```python
from build123d import *

# Parameters (mm, degrees)
F0_R     = 2.8256485239
F0_R_2   = 3.5765465122
F0_R_3   = 2.7439429232
F0_R_4   = 3.3466336439
F0_R_5   = 3.4276298102
F0_R_6   = 3.6294104123
F0_R_7   = 2.635041669
F0_R_8   = 2.702327646
F0_R_9   = 2.972249944
F0_R_10  = 2.6404432644
F0_R_11  = 2.6241403427
F0_R_12  = 2.7159497561
F0_R_13  = 2.2390207397
F0_R_14  = 2.2607819858
F0_R_15  = 1.9741758504
F0_R_16  = 2.1219308593
F0_R_17  = 1.8827842167
F0_R_18  = 1.845321618
F0_R_19  = 1.9213841029
F1_DEPTH = 25


with BuildPart() as f1:
    # F0 (on Front) → F1 (new body)
    with BuildSketch(Plane.XZ):
        with BuildLine():
            ThreePointArc((24.5960952758, -4.4757230907), (24.8988190673, -2.2469555075), (25, 0))
            ThreePointArc((25, 0), (24.9769503507, 1.073289886), (24.9078439057, 2.1446006555))
            ThreePointArc((24.9078439057, 2.1446006555), (0.5208838947, 24.9945730103), (-24.7968706797, 3.1804409279))
            ThreePointArc((-24.7968706797, 3.1804409279), (-23.1514874221, -9.4344385176), (-15.5110739298, -19.6062894384))
            ThreePointArc((-15.5110739298, -19.6062894384), (-13.7709472228, -14.2438804489), (-9.2095510788, -17.5570566207))
            ThreePointArc((-9.2095510788, -17.5570566207), (-10.6398306506, -20.3713740635), (-13.7563172666, -20.8749547368))
            ThreePointArc((-13.7563172666, -20.8749547368), (-7.1807427047, -23.9465432622), (0, -25))
            ThreePointArc((0, -25), (13.7903970721, -20.8524566561), (23.0050925772, -9.7859958876))
            ThreePointArc((23.0050925772, -9.7859958876), (16.860220208, -5.0514647504), (24.5960952758, -4.4757230907))
        make_face()
        with Locations((-7.0527321659, -21.0157949477)):
            Circle(F0_R, mode=Mode.SUBTRACT)
        with Locations((-18.0755164474, -11.404263787)):
            Circle(F0_R_2, mode=Mode.SUBTRACT)
        with Locations((-21.2986432016, -5.0265877508)):
            Circle(F0_R_3, mode=Mode.SUBTRACT)
        Polygon((4.266737029, -20.0934484601), (0, -25), (-2.6190390345, -20.0934484601), align=None, mode=Mode.SUBTRACT)
        with Locations((9.209163487, -19.5164699107)):
            Circle(F0_R_4, mode=Mode.SUBTRACT)
        with Locations((14.8604605347, -15.1914991438)):
            Circle(F0_R_5, mode=Mode.SUBTRACT)
        with BuildLine():
            Line((-18.9121421427, -0.7938772906), (-24.7968706797, 3.1804409279))
            Line((-24.7968706797, 3.1804409279), (-19.3468905014, 5.0684465431))
            ThreePointArc((-19.3468905014, 5.0684465431), (-21.9186154294, 11.469459375), (-15.5548330751, 8.8069401681))
            ThreePointArc((-15.5548330751, 8.8069401681), (-16.5182971087, 6.3016908172), (-18.9121421427, 5.0875890061))
            Line((-18.9121421427, 5.0875890061), (-18.9121421427, -0.7938772906))
        make_face(mode=Mode.SUBTRACT)
        with Locations((-7.0253848098, 20.105432719)):
            Circle(F0_R_6, mode=Mode.SUBTRACT)
        with BuildLine():
            Line((19.5046194307, 4.8279847044), (24.9078439057, 2.1446006555))
            Line((24.9078439057, 2.1446006555), (18.717167899, 0))
            Line((18.717167899, 0), (18.717167899, 4.7704775792))
            ThreePointArc((18.717167899, 4.7704775792), (17.4488389654, 5.1069570809), (16.4242905584, 5.9268212774))
            ThreePointArc((16.4242905584, 5.9268212774), (17.1998275024, 3.0083990244), (17.4609430101, 0))
            ThreePointArc((17.4609430101, 0), (-6.6059492578, -16.1631050607), (-12.4625227562, 12.2298837833))
            ThreePointArc((-12.4625227562, 12.2298837833), (-16.8312529103, 17.4566617233), (-10.3065616702, 15.4987508431))
            ThreePointArc((-10.3065616702, 15.4987508431), (-10.4242678564, 14.5913936768), (-10.7695943307, 13.7441030538))
            ThreePointArc((-10.7695943307, 13.7441030538), (-2.5101792072, 17.2795697617), (6.4137999623, 16.2403109836))
            ThreePointArc((6.4137999623, 16.2403109836), (5.9393579148, 21.9051948536), (10.9397131516, 19.2010402679))
            ThreePointArc((10.9397131516, 19.2010402679), (9.558784183, 16.551960716), (6.5962795119, 16.1670537638))
            ThreePointArc((6.5962795119, 16.1670537638), (9.4231129686, 14.6999820674), (11.9364463054, 12.7438526513))
            ThreePointArc((11.9364463054, 12.7438526513), (14.1879258767, 18.3986934482), (19.0337079573, 14.7156538442))
            ThreePointArc((19.0337079573, 14.7156538442), (17.0365778867, 11.3571292026), (13.1320353046, 11.5080050208))
            ThreePointArc((13.1320353046, 11.5080050208), (14.5572332623, 9.6421725015), (15.7192265164, 7.6020029287))
            ThreePointArc((15.7192265164, 7.6020029287), (18.7083751896, 11.1226574982), (22.0615752041, 7.9468004405))
            ThreePointArc((22.0615752041, 7.9468004405), (21.3406257649, 5.9303038237), (19.5046194307, 4.8279847044))
        make_face(mode=Mode.SUBTRACT)
        Polygon((3.975788597, 19.6694843471), (-2.6190390345, 19.6694843471), (0, 24.2276750505), align=None, mode=Mode.SUBTRACT)
        with BuildLine():
            ThreePointArc((23.0050925772, -9.7859958876), (23.9482362722, -7.1750943862), (24.5960952758, -4.4757230907))
            ThreePointArc((24.5960952758, -4.4757230907), (16.860220208, -5.0514647504), (23.0050925772, -9.7859958876))
        make_face()
        with Locations((20.8382867277, -6.2433271669)):
            Circle(F0_R_7, mode=Mode.SUBTRACT)
        with BuildLine():
            ThreePointArc((11.9364463054, 12.7438526513), (12.5494630323, 12.1406551883), (13.1320353046, 11.5080050208))
            ThreePointArc((13.1320353046, 11.5080050208), (17.0365778867, 11.3571292026), (19.0337079573, 14.7156538442))
            ThreePointArc((19.0337079573, 14.7156538442), (14.1879258767, 18.3986934482), (11.9364463054, 12.7438526513))
        make_face()
        with Locations((15.2111686766, 14.7156538442)):
            Circle(F0_R_8, mode=Mode.SUBTRACT)
        with BuildLine():
            ThreePointArc((-15.5548330751, 8.8069401681), (-21.9186154294, 11.469459375), (-19.3468905014, 5.0684465431))
            Line((-19.3468905014, 5.0684465431), (-18.9121421427, 5.2190539427))
            Line((-18.9121421427, 5.2190539427), (-18.9121421427, 5.0875890061))
            ThreePointArc((-18.9121421427, 5.0875890061), (-16.5182971087, 6.3016908172), (-15.5548330751, 8.8069401681))
        make_face()
        with Locations((-19.2937050015, 8.8069401681)):
            Circle(F0_R_9, mode=Mode.SUBTRACT)
        with Locations((-7.0253848098, 20.105432719)):
            Circle(F0_R_6)
        with Locations((-7.0253848098, 20.105432719)):
            Circle(F0_R_10, mode=Mode.SUBTRACT)
        with Locations((-18.0755164474, -11.404263787)):
            Circle(F0_R_2)
        with Locations((-18.0755164474, -11.404263787)):
            Circle(F0_R_11, mode=Mode.SUBTRACT)
        with BuildLine():
            ThreePointArc((-10.3065616702, 15.4987508431), (-16.8312529103, 17.4566617233), (-12.4625227562, 12.2298837833))
            ThreePointArc((-12.4625227562, 12.2298837833), (-11.6407057812, 13.0145495395), (-10.7695943307, 13.7441030538))
            ThreePointArc((-10.7695943307, 13.7441030538), (-10.4242678564, 14.5913936768), (-10.3065616702, 15.4987508431))
        make_face()
        with Locations((-13.8626694679, 15.4987508431)):
            Circle(F0_R_12, mode=Mode.SUBTRACT)
        with BuildLine():
            ThreePointArc((-9.2095510788, -17.5570566207), (-13.7709472228, -14.2438804489), (-15.5110739298, -19.6062894384))
            ThreePointArc((-15.5110739298, -19.6062894384), (-14.6474374814, -20.2596291977), (-13.7563172666, -20.8749547368))
            ThreePointArc((-13.7563172666, -20.8749547368), (-10.6398306506, -20.3713740635), (-9.2095510788, -17.5570566207))
        make_face()
        with Locations((-12.6935141161, -17.5570566207)):
            Circle(F0_R_13, mode=Mode.SUBTRACT)
        with Locations((14.8604605347, -15.1914991438)):
            Circle(F0_R_5)
        with Locations((14.8604605347, -15.1914991438)):
            Circle(F0_R_14, mode=Mode.SUBTRACT)
        with Locations((9.209163487, -19.5164699107)):
            Circle(F0_R_4)
        with Locations((9.209163487, -19.5164699107)):
            Circle(F0_R_15, mode=Mode.SUBTRACT)
        with BuildLine():
            ThreePointArc((6.4137999623, 16.2403109836), (6.5051428606, 16.2039392484), (6.5962795119, 16.1670537638))
            ThreePointArc((6.5962795119, 16.1670537638), (9.558784183, 16.551960716), (10.9397131516, 19.2010402679))
            ThreePointArc((10.9397131516, 19.2010402679), (5.9393579148, 21.9051948536), (6.4137999623, 16.2403109836))
        make_face()
        with Locations((7.7083422802, 19.2010402679)):
            Circle(F0_R_16, mode=Mode.SUBTRACT)
        with BuildLine():
            Line((18.717167899, 5.2190539427), (19.5046194307, 4.8279847044))
            ThreePointArc((19.5046194307, 4.8279847044), (21.3406257649, 5.9303038237), (22.0615752041, 7.9468004405))
            ThreePointArc((22.0615752041, 7.9468004405), (18.7083751896, 11.1226574982), (15.7192265164, 7.6020029287))
            ThreePointArc((15.7192265164, 7.6020029287), (16.0935695505, 6.7735920991), (16.4242905584, 5.9268212774))
            ThreePointArc((16.4242905584, 5.9268212774), (17.4488389654, 5.1069570809), (18.717167899, 4.7704775792))
            Line((18.717167899, 4.7704775792), (18.717167899, 5.2190539427))
        make_face()
        with Locations((18.8810285181, 7.9468004405)):
            Circle(F0_R_17, mode=Mode.SUBTRACT)
        with Locations((-7.0527321659, -21.0157949477)):
            Circle(F0_R)
        with Locations((-7.0527321659, -21.0157949477)):
            Circle(F0_R_18, mode=Mode.SUBTRACT)
        with Locations((-21.2986432016, -5.0265877508)):
            Circle(F0_R_3)
        with Locations((-21.2986432016, -5.0265877508)):
            Circle(F0_R_19, mode=Mode.SUBTRACT)
        with BuildLine():
            Line((-19.3468905014, 5.0684465431), (-24.7968706797, 3.1804409279))
            Line((-24.7968706797, 3.1804409279), (-18.9121421427, -0.7938772906))
            Line((-18.9121421427, -0.7938772906), (-18.9121421427, 5.0875890061))
            ThreePointArc((-18.9121421427, 5.0875890061), (-19.1292375855, 5.0716873319), (-19.3468905014, 5.0684465431))
        make_face()
        Polygon((-19.7024215013, 4.2425552383), (-19.7024215013, 0.5726945819), (-23.453835398, 3.1415971462), align=None, mode=Mode.SUBTRACT)
        Polygon((-2.6190390345, -20.0934484601), (0, -25), (4.266737029, -20.0934484601), align=None)
        Polygon((0, -23.921410939), (-1.2212268775, -21.310839802), (2.2701525595, -21.310839802), align=None, mode=Mode.SUBTRACT)
        with BuildLine():
            Line((18.717167899, 0), (24.9078439057, 2.1446006555))
            Line((24.9078439057, 2.1446006555), (19.5046194307, 4.8279847044))
            ThreePointArc((19.5046194307, 4.8279847044), (19.1126850593, 4.774701377), (18.717167899, 4.7704775792))
            Line((18.717167899, 4.7704775792), (18.717167899, 0))
        make_face()
        Polygon((23.5085282475, 2.1446006555), (19.1881656647, 0.9002434672), (19.1881656647, 4.50054463), align=None, mode=Mode.SUBTRACT)
        Polygon((0, 24.2276750505), (-2.6190390345, 19.6694843471), (3.975788597, 19.6694843471), align=None)
        Polygon((2.4991026148, 20.1859623194), (-1.6240375116, 20.1859623194), (0, 23.2999436557), align=None, mode=Mode.SUBTRACT)
        with BuildLine():
            ThreePointArc((18.717167899, 4.7704775792), (19.1126850593, 4.774701377), (19.5046194307, 4.8279847044))
            Line((19.5046194307, 4.8279847044), (18.717167899, 5.2190539427))
            Line((18.717167899, 5.2190539427), (18.717167899, 4.7704775792))
        make_face()
        with BuildLine():
            Line((-18.9121421427, 5.2190539427), (-19.3468905014, 5.0684465431))
            ThreePointArc((-19.3468905014, 5.0684465431), (-19.1292375855, 5.0716873319), (-18.9121421427, 5.0875890061))
            Line((-18.9121421427, 5.0875890061), (-18.9121421427, 5.2190539427))
        make_face()
    extrude(amount=F1_DEPTH)


solid = f1.part
```
Can you work these out from the model? Positions are in its coordinate system, mm. Give positions to 0.01 mm unless a question says otherwise; leave off trailing zeros. Order: outer loops, then holes, each group sorted by start corner. A loop starts at its lowest first (then second) coordinate and runs counter-clockwise, first axis right, second up. Notation, with made-up numbers: (-15.75, -33.5) - (41.25, -33.5) arc R13 cw to (41.25, -23.5) - close; hole circle Ø9 at (9, -32.75). An arc over 180 degrees is marked (long way). Use a Markdown table: item, result. Add a question column.
Q1. Please list where these lines run through material, in increasing order: line 1 along X through (y, z) = (-5.5, -10); line 2 along Z through (x, y) = (22.5, -8.25); line 3 along Z through (x, y) = (-13, -20.25) (3 decimals).
Q2. I'm going to push flat-ended pins straight in: pin 1 (3 mm diameter, centred on y = -15, z = 2.5, fed in from +X); pin 2 (1 mm diameter, centred on x = 10.5, y = -22, fed in from +Z); pin 3 (8 mm diameter, centred on x = -4.5, y = -13, fed in from +Z) (3 decimals). Where does each tip first touch, or does it pass through?
Q3. If we section it at D-D on y = -18.5: Count the separate pieces of the cut face and the enclosed holes in it, plus the area to 3 significant figures.
Q4. If we section it at B-B on z = -2.5: Write out the boundary of the cut face in (x, y), plus the area to 3 significant figures.
Q5. If we mould it in two halves opening along X, with no side actions, what happens to faces 1 (the cylindrical face through (10.12, -12.32, -21.27)), 2 (the flat face through (-6, -25, 17))? For each: released by +X, released by -X, zero draft, split by the parting line, or undercut.
Q6. If we section it at C-C on z = -8: Write out the boundary of the cut face in (x, y), plus the area to 3 significant figures.
Q7. If we section it at A-A on x = 3.5: Write out the boundary of the cut face in (y, z), plus the area to 3 significant figures.
Answers follow:
| question | item | result |
|---|---|---|
| 1 | line 1 | x = -22.91 to -20.29, -15.86 to -14.31, 14.31 to 22.91 |
| 1 | line 2 | z = -10.9 to -8.29, -4.2 to 1.85, 2.69 to 10.9 |
| 1 | line 3 | z = -21.354 to -19.775, -15.339 to -11.657, 11.657 to 12.923, 18.074 to 21.354 |
| 2 | pin 1 | stops at x = 24.98 |
| 2 | pin 2 | stops at z = 22.91 |
| 2 | pin 3 | stops at z = 24.995 |
| 3 | separate pieces | 1 |
| 3 | enclosed holes | 18 |
| 3 | area | 749 mm^2 |
| 4 | outline | (-24.87, -25) - (-17.28, -25) - (-17.28, 0) - (-24.87, 0) - close; (17.28, -25) - (24.87, -25) - (24.87, 0) - (17.28, 0) - close |
| 4 | area | 380 mm^2 |
| 5 | face 1 | undercut |
| 5 | face 2 | zero draft |
| 6 | outline | (-23.69, -25) - (-15.52, -25) - (-15.52, 0) - (-23.69, 0) - close; (15.52, -25) - (18.87, -25) - (18.87, 0) - (15.52, 0) - close; (22.8, -25) - (23.69, -25) - (23.69, 0) - (22.8, 0) - close |
| 6 | area | 310 mm^2 |
| 7 | outline | (-25, -24.75) - (0, -24.75) - (0, -17.11) - (-25, -17.11) - close; (-25, 17.11) - (0, 17.11) - (0, 24.75) - (-25, 24.75) - close |
| 7 | area | 382 mm^2 |
